Geometry: see drawing. Coordinates: mm, zero at the bounding-box minimum. Coordinates: 2 decimals unless noted, no trailing zeros. Loops run counter-clockwise (first coordinate to the right, second up) from the corner with the lowest first, then second, coordinate; pieces in that order, holes last. Notation, with made-up numbers: (84.25, -19.5) - (106.25, -19.5) arc R16 ccw to (106.25, -14.5) - close; hole circle Ø11 at (47, 12.5). An arc over 180 degrees is marked (long way). Write each question's results on one line, items separated by ' | '. Start each with the question number.
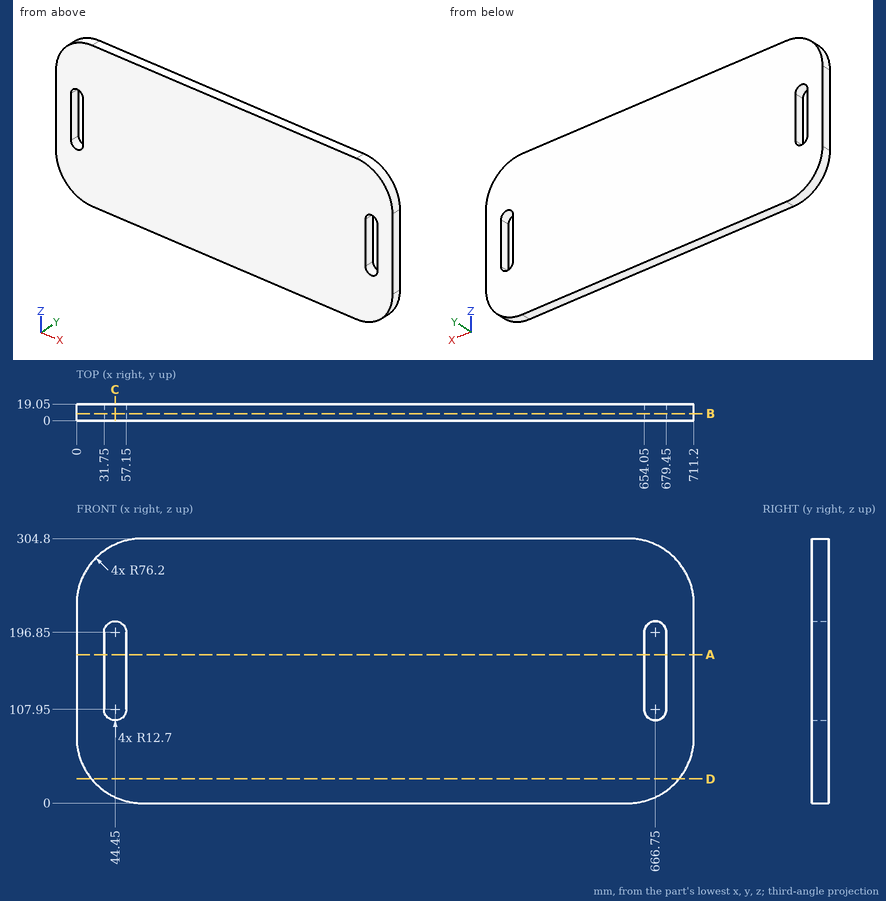
1) Pin query (flat end, axial travel): pin 1 Ø2 at (y, z) = (15.5, 74) entering from +X; pin 2 Ø8 at (y, z) = (15.5, 252) entering from +X; pin 3 Ø1 at (y, z) = (10, 67) entering from +X. Return the tip coordinate at first contact, or that it passes through.
2) Section query A-A on z = 171. Output: boundary loops of the cut face in (x, y).
3) Section query D-D on z = 28. Output: boundary loops of the cut face in (x, y), and give its area (3 significant figures).
4) Section query B-B on y = 8. Output: boundary loops of the cut face in (x, z), and give its area (3 significant figures).
5) Material intervals for line 1 (X direction, y = 7.5, z = 177.5); line 2 (X direction, y = 16.25, z = 229); line 3 (Z direction, x = 666, y = 17), sorted ascending. Write a range as [from, to].
6) Section query C-C on x = 44.45. Output: boundary loops of the cut face in (y, z).
Returned:
1) pin 1: stops at x = 711.19 | pin 2: stops at x = 708.69 | pin 3: stops at x = 710.7
2) outline: (0, 0) - (31.75, 0) - (31.75, 19.05) - (0, 19.05) - close; (57.15, 0) - (654.05, 0) - (654.05, 19.05) - (57.15, 19.05) - close; (679.45, 0) - (711.2, 0) - (711.2, 19.05) - (679.45, 19.05) - close
3) outline: (17.18, 0) - (694.02, 0) - (694.02, 19.05) - (17.18, 19.05) - close | area: 12,900 mm²
4) outline: (0, 76.2) arc R76.2 ccw to (76.2, 0) - (635, 0) arc R76.2 ccw to (711.2, 76.2) - (711.2, 228.6) arc R76.2 ccw to (635, 304.8) - (76.2, 304.8) arc R76.2 ccw to (0, 228.6) - close; hole (31.75, 107.95) arc R12.7 ccw to (57.15, 107.95) - (57.15, 196.85) arc R12.7 ccw to (31.75, 196.85) - close; hole (654.05, 107.95) arc R12.7 ccw to (679.45, 107.95) - (679.45, 196.85) arc R12.7 ccw to (654.05, 196.85) - close | area: 206,000 mm²
5) line 1: x = [0, 31.75], [57.15, 654.05], [679.45, 711.2] | line 2: x = [0, 711.2] | line 3: z = [6.59, 95.27], [209.53, 298.21]
6) outline: (0, 6.93) - (19.05, 6.93) - (19.05, 95.25) - (0, 95.25) - close; (0, 209.55) - (19.05, 209.55) - (19.05, 297.87) - (0, 297.87) - close
